Part model, mm, in its own coordinate system. Face numbers are marked on the shaded views. A direction names the side the tool comes from. Give positions to 0.01 mm unless a question says otherwise; leave off trailing zeros. Loops run counter-clockwise (first coordinate to the right, second up) from the corner with the lowest first, then second, coordinate; pieces in that order, holes last. Notation, with made-up numbers: (19, -0.5) -> (56, -0.5) arc R9 cw to (56, 4.5) -> close; hole circle Ø4 at (-11.75, 0). An arc over 180 degrees is marked (long way). One line per question, with ' | ' between items.
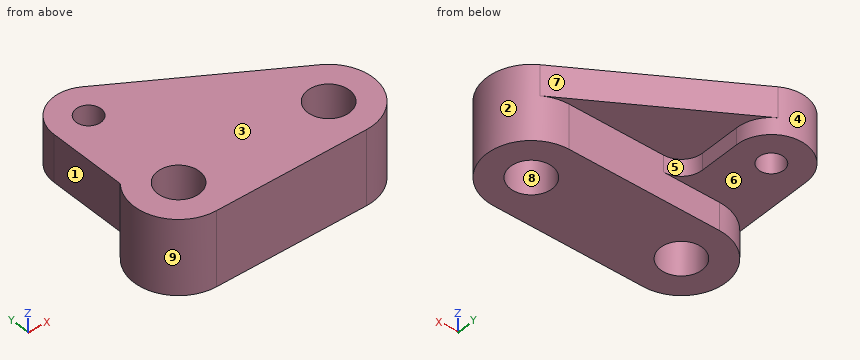
```python
from build123d import *

# Parameters (mm, degrees)
SKETCH1_R           = 15
BOSS_EXTRUDE1_DEPTH = 27
BOSS_EXTRUDE3_DEPTH = 34
SKETCH2_3_R         = 9
CUT_EXTRUDE1_DEPTH  = 34
FILLET1_R           = 15
BOSS_EXTRUDE4_DEPTH = 22


with BuildPart() as part:
    # Sketch1 → Boss-Extrude1 (new, symmetric)
    with BuildSketch(Plane.XY):
        with BuildLine():
            Line((-108, 32), (0, 32))
            ThreePointArc((0, 32), (32, 0), (0, -32))
            Line((0, -32), (-108, -32))
            ThreePointArc((-108, -32), (-140, 0), (-108, 32))
        make_face()
        Circle(SKETCH1_R, mode=Mode.SUBTRACT)
        with Locations((-108, 0)):
            Circle(SKETCH1_R, mode=Mode.SUBTRACT)
    extrude(amount=BOSS_EXTRUDE1_DEPTH, both=True)

    # Sketch2 → Boss-Extrude3 (add)
    with BuildSketch(Plane.XY.offset(27)):
        with BuildLine():
            Line((-83, 76), (-83, 32))
            Line((-83, 32), (-108, 32))
            ThreePointArc((-108, 32), (-121.870841731, 28.837471278), (-133, 19.974984355))
            Line((-133, 19.974984355), (-133, 76))
            ThreePointArc((-133, 76), (-108, 101), (-83, 76))
        make_face()
    extrude(amount=-BOSS_EXTRUDE3_DEPTH)

    # Sketch2_3 → Cut-Extrude1 (cut)
    with BuildSketch(Plane.XY.offset(27)):
        with Locations(Location((-108, 76, 0), (0, 0, 180))):
            Circle(SKETCH2_3_R)
    extrude(amount=-CUT_EXTRUDE1_DEPTH, mode=Mode.SUBTRACT)

    # Fillet1
    fillet1_edges = [part.edges().sort_by_distance(p)[0] for p in [
        (-83, 32, 10),
    ]]
    fillet(fillet1_edges, radius=FILLET1_R)

    # Sketch3 → Boss-Extrude4 (add)
    with BuildSketch(Plane.XY.offset(27)):
        with BuildLine():
            Line((-94.716606225, 97.17903326), (17.002744032, 27.109162572))
            ThreePointArc((17.002744032, 27.109162572), (8.846095118, 30.752993369), (0, 32))
            Line((0, 32), (-68, 32))
            ThreePointArc((-68, 32), (-78.606601718, 36.393398282), (-83, 47))
            Line((-83, 47), (-83, 76))
            ThreePointArc((-83, 76), (-86.124387501, 88.101965865), (-94.716606225, 97.17903326))
        make_face()
    extrude(amount=-BOSS_EXTRUDE4_DEPTH)


solid = part.part
```
1) Drill centre lines: line 1 (Y direction, x = -108, z = 13.5); line 2 (X direction, y = -12.5, z = 6.5); line 3 (X direction, y = 76, z = 3.5). Where is each one in solid material? Low to high.
Found:
line 1: -32 to -15, 15 to 67, 85 to 101 | line 2: -137.46 to -116.29, -99.71 to -8.29, 8.29 to 29.46 | line 3: -133 to -117, -99 to -83
2) Pin check, flat tips, straight feed: P1, Ø5, axis at y = 21, z = -16, coming from the +X side; P2, Ø10, axis at y = -7, z = -21.5, coming from the +X side; P3, Ø17, axis at y = 61, z = 16, coming from the -X side. Stop position of each tip, or through.
Found:
P1: x = 26.11 | P2: x = 31.94 | P3: x = -133
3) Saw through at B-B (x = -105.5). Give the cut face in (y, z), and give its area (3 significant figures).
Found:
outline: (-32, -27) -> (-14.79, -27) -> (-14.79, 27) -> (-32, 27) -> close; (14.79, -27) -> (32, -27) -> (32, -7) -> (67.35, -7) -> (67.35, 27) -> (14.79, 27) -> close; (84.65, -7) -> (100.87, -7) -> (100.87, 27) -> (84.65, 27) -> close | area: 3,610 mm2
4) Saw through at C-C (y = 70.5). Give the cut face in (x, z).
Found:
outline: (-133, -7) -> (-115.12, -7) -> (-115.12, 27) -> (-133, 27) -> close; (-100.88, -7) -> (-83, -7) -> (-83, 5) -> (-52.18, 5) -> (-52.18, 27) -> (-100.88, 27) -> close
5) Tool access for the marked faces 1, 2, 3, 4 and 5: list every direction of +Z, -Z, +X, -X, +Y, -Y with a clear straight run to the whole face (end or side of a thin tool).
Found:
face 1: +Z, -Z, -X, +Y | face 2: -Z, +X | face 3: +Z, +X, -X, +Y, -Y | face 4: -Z, +Y | face 5: -Z, +X, +Y
6) Saw through at A-A (y = 0). Give the cut face in (x, z).
Found:
outline: (-140, -27) -> (-123, -27) -> (-123, 27) -> (-140, 27) -> close; (-93, -27) -> (-15, -27) -> (-15, 27) -> (-93, 27) -> close; (15, -27) -> (32, -27) -> (32, 27) -> (15, 27) -> close
7) Pull direction X, two halves, no side cores. Call the marked faces 6, 7, 8 and 9: pulls with the +X half, pulls with the -X half, needs draft (parallel to the pull), parting line crosses it, or undercut.
Found:
face 6: needs draft | face 7: pulls with the +X half | face 8: undercut | face 9: pulls with the -X half
8) Saw through at D-D (y = 88). Give the cut face in (x, z).
Found:
outline: (-129.93, -7) -> (-86.07, -7) -> (-86.07, 5) -> (-80.08, 5) -> (-80.08, 27) -> (-129.93, 27) -> close
